Geometry: final body of the model. Coordinates: model frame, mm. Face numbers are marked on the shaded views. A direction names the side the tool comes from. Coordinates: 2 decimals unless noted, no trailing zeros. Order: outer loops, then holes, each group sorted by start corner. A loop starts at its lowest first (then second) coordinate and runs counter-clockwise, first axis right, second up. Notation, with made-up numbers: M 32,48 L 43,48 A14 ccw 43,66 Z; hole C 61.25,-12 d7. An arc over 180 degrees is marked long. Use CSV: the item, a comma, the result in double quotes. Start each with the question number.
1. Section query C-C on y = 67. Return the cut outline in (x, z), and give its area (3 significant figures).
2. First-contact query: P1, Ø11.5, axis at x = 148, y = 71, coming from the -Z side; P2, Ø12, axis at x = 60, y = 62, coming from the -Z side; P3, Ø6, axis at x = -104.5, z = 120, coming from the +Y side. Flat tips, straight axial feed; report the tip coordinate or a pass-through.
3. Pull-direction query (X, two-part tool) for the marked faces 1, 2 and 3; classes: pulls with the +X half, pulls with the -X half, needs draft (parallel to the pull), parting line crosses it, or undercut.
4. Material intervals for line 1 (Y direction, x = 10, z = 85.5); line 2 (Z direction, x = 72, y = 84); line 3 (X direction, y = 68, z = 136), sorted ascending.
5. Section query B-B on z = 22. Return the cut outline in (x, y), and give its area (3 significant figures).
6. Set-up query: the marked faces 4 and 5. Return all of +Z, -Z, +X, -X, +Y, -Y with unobstructed straight access to the full face (end or side cutting, diameter ignored); none if empty.
7. Section query D-D on z = 130.5. Return the cut outline in (x, y).
8. Section query A-A on x = -94.5. Return the cut outline in (y, z).
from build123d import *

# Parameters (mm, degrees)
BOSS_EXTRU_1_DEPTH           = 5.5
BOSS_EXTRU_2_DEPTH           = 96
ENL_V_MAT_EXTRU_1_DEPTH      = 39
ENL_V_MAT_EXTRU_1_DEPTH_BACK = 37
ESQUISSE3_W                  = 197.227924694
ESQUISSE3_H                  = 161.841973662
BOSS_EXTRU_3_DEPTH           = 5.5


with BuildPart() as part:
    # Esquisse1 → Boss.-Extru.1 (new body)
    with BuildSketch(Plane(origin=(0, 0, 0), x_dir=(-1, 0, 0), z_dir=(0, 1, 0))):
        Polygon((-151.846153846, 122.087912088), (-125.490601914, 152.208542868), (125.490601914, 152.208542868), (151.846153846, 122.087912088), (151.846153846, -122.087912088), (-151.846153846, -122.087912088), align=None)
    extrude(amount=BOSS_EXTRU_1_DEPTH)

    # Esquisse2 → Boss.-Extru.2 (add)
    with BuildSketch(Plane(origin=(0, 5.5, 0), x_dir=(1, 0, 0), z_dir=(0, 1, 0))):
        Polygon((-151.846153846, -122.087912088), (-140.09050176, -122.087912088), (-125.734949828, -137.938542868), (125.490601914, -137.938542868), (141.341232694, -122.087912088), (151.846153846, -122.087912088), (125.490601914, -152.208542868), (-125.490601914, -152.208542868), align=None)
    extrude(amount=BOSS_EXTRU_2_DEPTH)

    # Esquisse3 → Enlèv. mat.-Extru.1 (cut, two sides: drawn at the far end of the back side and taken through both)
    with BuildSketch(Plane.XZ.offset(-ENL_V_MAT_EXTRU_1_DEPTH_BACK)):
        Rectangle(ESQUISSE3_W, ESQUISSE3_H)
    extrude(amount=ENL_V_MAT_EXTRU_1_DEPTH + ENL_V_MAT_EXTRU_1_DEPTH_BACK, mode=Mode.SUBTRACT)

    # Esquisse4 → Boss.-Extru.3 (add)
    with BuildSketch(Plane.XZ):
        Polygon((-10.738571279, 80.920986831), (10.738571279, 80.920986831), (10.738571279, 10), (98.613962347, 10), (98.613962347, -10), (10.738571279, -10), (10.738571279, -80.920986831), (-10.738571279, -80.920986831), (-10.738571279, -10), (-98.613962347, -10), (-98.613962347, 10), (-10.738571279, 10), align=None)
    extrude(amount=-BOSS_EXTRU_3_DEPTH)


solid = part.part
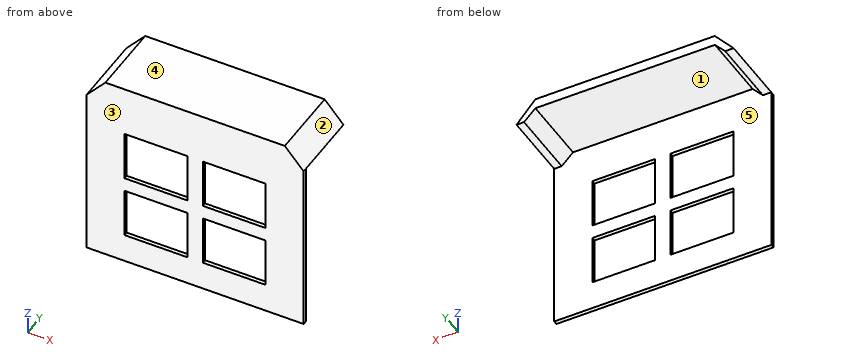
Results list:
1,outline,"M -151.85,122.09 L -140.09,122.09 L -125.73,137.94 L 125.49,137.94 L 141.34,122.09 L 151.85,122.09 L 125.49,152.21 L -125.49,152.21 Z"
1,area,"4,130 mm²"
2,P1,"stops at z = 122.09"
2,P2,"stops at z = 137.94"
2,P3,"stops at y = 5.5"
3,face 1,"undercut"
3,face 2,"pulls with the +X half"
3,face 3,"needs draft"
4,line 1,"y = 0 to 5.5"
4,line 2,"z = 137.94 to 152.21"
4,line 3,"x = -139.67 to -127.49, 127.43 to 139.67"
5,outline,"M -151.85,0 L -98.61,0 L -98.61,5.5 L -151.85,5.5 Z; M -10.74,0 L 10.74,0 L 10.74,5.5 L -10.74,5.5 Z; M 98.61,0 L 151.85,0 L 151.85,5.5 L 98.61,5.5 Z"
5,area,"704 mm²"
6,face 4,"+Z, +X, -X, +Y, -Y"
6,face 5,"-Z, +Y"
7,outline,"M -144.49,0 L 144.49,0 L 144.49,101.5 L 132.93,101.5 L 132.93,5.5 L -132.47,5.5 L -132.47,101.5 L -144.49,101.5 Z"
8,outline,"M 0,-122.09 L 5.5,-122.09 L 5.5,-80.92 L 0,-80.92 Z; M 0,-10 L 5.5,-10 L 5.5,10 L 0,10 Z; M 0,80.92 L 5.5,80.92 L 5.5,137.94 L 101.5,137.94 L 101.5,152.21 L 0,152.21 Z"
